```python
from build123d import *

# Parameters (mm, degrees)
BOX101_W     = 140
BOX101_H     = 80
BOX101_DEPTH = 190
BOX102_W     = 140
BOX102_H     = 80
BOX102_DEPTH = 190
BOX103_W     = 195
BOX103_H     = 140
BOX103_DEPTH = 190


with BuildPart() as cube073:
    # Box101 → Box101 (new body)
    with BuildSketch(Plane(origin=(220, 30, 0), x_dir=(1, 0, 0), z_dir=(0, 0, 1))):
        with Locations((70, 40)):
            Rectangle(BOX101_W, BOX101_H)
    extrude(amount=BOX101_DEPTH)


with BuildPart() as fusion017:
    # Box102 → Box102 (new body)
    with BuildSketch(Plane(origin=(30, 30, 0), x_dir=(1, 0, 0), z_dir=(0, 0, 1))):
        with Locations((70, 40)):
            Rectangle(BOX102_W, BOX102_H)
    extrude(amount=BOX102_DEPTH)

    # Fusion017: union Cube073
    add(cube073.part)


with BuildPart() as obj1:
    # Box103 → Box103 (new body)
    with BuildSketch(Plane.XY):
        with Locations((97.5, 70)):
            Rectangle(BOX103_W, BOX103_H)
    extrude(amount=BOX103_DEPTH)

    # Cut012: cut Fusion017
    add(fusion017.part, mode=Mode.SUBTRACT)


with BuildPart() as obj1_1:
    # Cut012 placement: moved
    add(obj1.part.moved(Location((825, 445, -590))))


solid = obj1_1.part
```
CAD build for the part. Positions are in the model's coordinates, mm. A direction names the side the tool comes from. Coordinates: 2 decimals unless noted, no trailing zeros. Order: outer loops, then holes, each group sorted by start corner. A loop starts at its lowest first (then second) coordinate and runs counter-clockwise, first axis right, second up. Notation, with made-up numbers: M -15.75,34.5 L 43.25,34.5 A31 ccw 43.25,62.5 Z; hole C 78,51 d4. An arc over 180 degrees is marked long. Answer as CSV lines item,"result".
1) Cut at B-B (x = 934). List the corners of the cut face in (y, z).
Verdict:
outline,"M 445,-590 L 475,-590 L 475,-400 L 445,-400 Z; M 555,-590 L 585,-590 L 585,-400 L 555,-400 Z"
2) Mould opens along X. For faces 1 (the flat face through (921, 469, -590)), 2 (the flat face through (825, 514, -496)), 3 (the flat face through (855, 514, -496)) say: released by +X, released by -X, zero draft, split by the parting line, or undercut.
Verdict:
face 1,"zero draft"
face 2,"released by -X"
face 3,"undercut"
3) Cut at C-C (y = 531.5). List the corners of the cut face in (x, z), then the cut area to 4 significant figures.
Verdict:
outline,"M 825,-590 L 855,-590 L 855,-400 L 825,-400 Z; M 995,-590 L 1020,-590 L 1020,-400 L 995,-400 Z"
area,"10,450 mm2"
4) Cut at A-A (z = -423.5). List the corners of the cut face in (x, y), then the cut area to 3 significant figures.
Verdict:
outline,"M 825,445 L 1020,445 L 1020,585 L 825,585 Z; hole M 855,475 L 995,475 L 995,555 L 855,555 Z"
area,"16,100 mm2"
5) Drill centre lines: L1, parallel to X at y = 493, z = -446.5; L2, parallel to Y at x = 893.5, z = -438. Where is each one in solid material? Low to high. Write a range as from..to.
Verdict:
L1,"825..855, 995..1020"
L2,"445..475, 555..585"
6) 3-axis set-ups, long thin cutter, end or side, ignore diameter. For faces 4 (the flat face through (924, 475, -496)), 5 (the flat face through (921, 469, -400)): which of +Z, -Z, +X, -X, +Y, -Y reach the whole face in a straight line?
Verdict:
face 4,"+Z, -Z"
face 5,"+Z, +X, -X, +Y, -Y"
